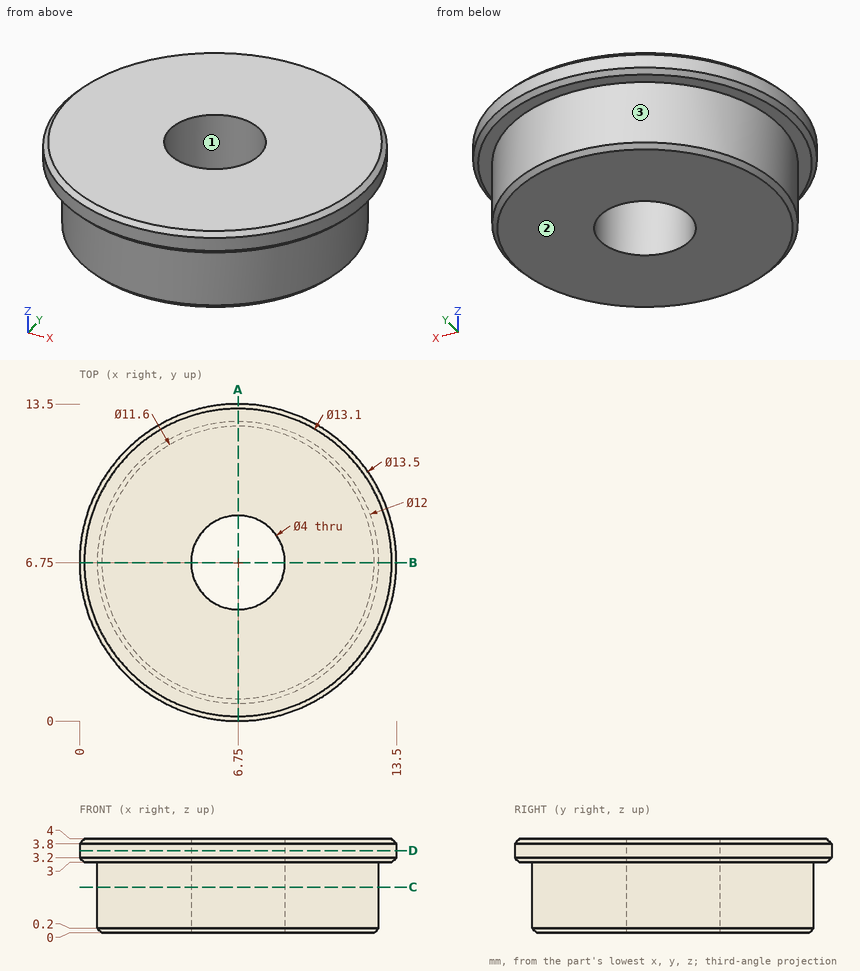
For this review, use the dimensioned drawing (mm, ordinates from the lowest corner) and the shaded views. Give positions to 0.01 mm unless a question says otherwise; leave off trailing zeros. Write each loop counter-clockwise with the first axis right and the second up, starting at its lowest first coordinate (ties: lowest second). Pieces come first, ordered by that corner, then holes.
(1) The part is to be moulded in two halves that separate along Y. For the marked faces 1, 2 and 3, say which applies: released by +Y, released by -Y, zero draft, split by the parting line, or undercut.
(2) To check wall thickness, follow L1, parallel to Y at x = 6.75, z = 2.6; L2, parallel to Y at x = 5.75, z = 0.5; L3, parallel to X at y = 7, z = 0.65. State the ranges of each line that lie inside material, in increasing order.
(3) For P1, Ø3, axis at x = 6.75, y = 6.75, coming from the -Z side; P2, Ø2, axis at y = 3.5, z = 1, coming from the -X side; P3, Ø2, axis at x = 8.5, z = 0.5, coming from the -Y side, all flat-tipped, find the tip position at first contact; note any pin that passes through.
(4) Consider section A-A, the plane x = 6.75. Give the boundary of the cut face in (y, z).
(5) Consider section D-D, the plane z = 3.5. Give the boundary of the cut face in (x, y), and give its area (3 significant figures).
(6) Consider section C-C, the plane z = 1.95. Give the boundary of the cut face in (x, y), and give its area (3 significant figures).
Returned:
1. face 1: undercut
1. face 2: zero draft
1. face 3: split by the parting line
2. L1: y = 0.75 to 4.75, 8.75 to 12.75
2. L2: y = 0.83 to 5.02, 8.48 to 12.67
2. L3: x = 0.76 to 4.77, 8.73 to 12.74
3. P1: passes through
3. P2: stops at x = 1.19
3. P3: stops at y = 0.8
4. outline: (0, 3.2) - (0.2, 3) - (0.75, 3) - (0.75, 0.2) - (0.95, 0) - (4.75, 0) - (4.75, 4) - (0.2, 4) - (0, 3.8) - close; (8.75, 0) - (12.55, 0) - (12.75, 0.2) - (12.75, 3) - (13.3, 3) - (13.5, 3.2) - (13.5, 3.8) - (13.3, 4) - (8.75, 4) - close
5. outline: circle Ø13.5 at (6.75, 6.75); hole circle Ø4 at (6.75, 6.75)
5. area: 131 mm2
6. outline: circle Ø12 at (6.75, 6.75); hole circle Ø4 at (6.75, 6.75)
6. area: 101 mm2
